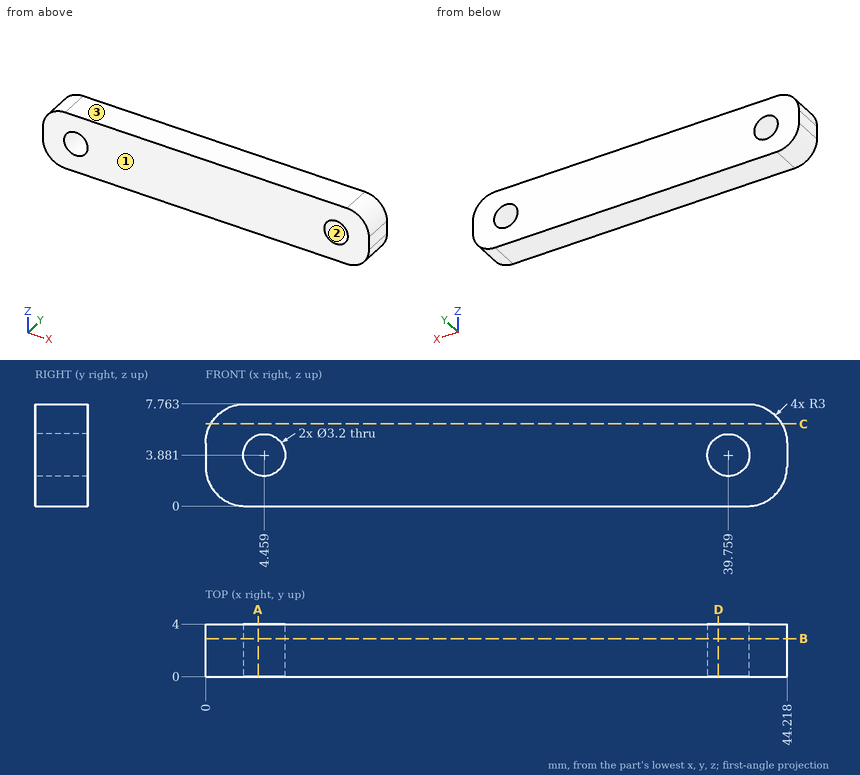
Source: three-view drawing plus pictorial views. Frame: mm from the lowest corner of the part. Coordinates: 2 decimals unless noted, no trailing zeros. Loops run counter-clockwise (first coordinate to the right, second up) from the corner with the lowest first, then second, coordinate; pieces in that order, holes last. Notation, with made-up numbers: (-13, 21.25) - (-7, 21.25) arc R25 cw to (-7, 56.25) - close; hole circle Ø3 at (53, 30). An arc over 180 degrees is marked (long way). Answer in a Markdown table with one row per item. Add a question column.
Item 1: Section query C-C on z = 6.25. Return the cut outline in (x, y) (1 decimal).
Item 2: Section query B-B on y = 2.9. Return the cut outline in (x, z).
Item 3: Section query A-A on x = 4. Return the cut outline in (y, z), then the cut area to 3 significant figures.
Item 4: Mould query, pull axis Z, two halves, no side actions, for the marked faces 1, 2 and 3. Classes: released by +Z, released by -Z, zero draft, split by the parting line, or undercut.
Item 5: Contact query for flat-ended pins moving along their axis: P1, Ø3, axis at x = 4.46, z = 3.88, coming from the -Y side; P2, Ø1.5, axis at y = 3, z = 6, coming from the -X side. Output: stop coordinate, or through.
Item 6: Section query D-D on x = 39. Return the cut outline in (y, z), then the cut area to 3 significant figures.
Item 7: Line query: line 1 along X through (y, z) = (0.95, 3.75) (1 decimal); line 2 along X through (y, z) = (3, 5.25) (1 decimal); line 3 along Z through (x, y) = (5, 0.95) (1 decimal). Output: solid intervals per line, ascending. Write a range as [from, to].
Recorded:
| question | item | result |
|---|---|---|
| 1 | outline | (0.4, 0) - (43.8, 0) - (43.8, 4) - (0.4, 4) - close |
| 2 | outline | (0, 3) arc R3 ccw to (3, 0) - (41.22, 0) arc R3 ccw to (44.22, 3) - (44.22, 4.76) arc R3 ccw to (41.22, 7.76) - (3, 7.76) arc R3 ccw to (0, 4.76) - close; hole circle Ø3.2 at (4.46, 3.88); hole circle Ø3.2 at (39.76, 3.88) |
| 3 | outline | (0, 0) - (4, 0) - (4, 2.35) - (0, 2.35) - close; (0, 5.41) - (4, 5.41) - (4, 7.76) - (0, 7.76) - close |
| 3 | area | 18.8 mm^2 |
| 4 | face 1 | zero draft |
| 4 | face 2 | undercut |
| 4 | face 3 | released by +Z |
| 5 | P1 | through |
| 5 | P2 | x = 0.04 |
| 6 | outline | (0, 0) - (4, 0) - (4, 2.47) - (0, 2.47) - close; (0, 5.29) - (4, 5.29) - (4, 7.76) - (0, 7.76) - close |
| 6 | area | 19.8 mm^2 |
| 7 | line 1 | [0, 2.9], [6.1, 38.2], [41.4, 44.2] |
| 7 | line 2 | [0, 3.6], [5.3, 38.9], [40.6, 44.2] |
| 7 | line 3 | [0, 2.4], [5.4, 7.8] |
